Autodesk Inventor part; units mm, degrees
ref_plane "YZ Plane" through (0, 0, 0) normal (1, 0, 0) x (0, 1, 0)
ref_plane "XZ Plane" through (0, 0, 0) normal (0, 1, 0) x (-1, 0, 0)
ref_plane "XY Plane" through (0, 0, 0) normal (0, 0, 1) x (1, 0, 0)
sketch "Sketch1" plane through (0, 0, 0) normal (0, 1, 0) x (-1, 0, 0)
  line L0 (12.5, -50) -> (-12.5, -50)
  line L1 (-12.5, -50) -> (-12.5, 10)
  line L2 (-12.5, 10) -> (12.5, 10)
  line L3 (12.5, 10) -> (12.5, -50)
  line L4 (12.5, 0) -> (-12.5, 0) construction
  line L5 (0, -50) -> (0, 10) construction
  circle A0 centre (7.5, 0) radius 1.6
  line L6 (12.5, 10) -> (146.5, 10)
  line L7 (146.5, 10) -> (146.5, -10)
  line L8 (146.5, -10) -> (12.5, -10)
  line L9 (12.5, -10) -> (12.5, 10)
  line L10 (146.5, 0) -> (12.5, 0) construction
  circle A1 centre (132.7538, 0) radius 2.5
  circle A2 centre (-7.5, 0) radius 1.6
  line L11 (12.5, -40) -> (-12.5, -40) construction
  circle A3 centre (7.5, -40) radius 2.5
  circle A4 centre (-7.5, -40) radius 2.5
  point P0 (0, 0)
  point P1 (0, 0)
  point P2 (12.5, -10)
  dimension "d0" = 3.2
  dimension "d1" = 15
  dimension "d3" = 10
  dimension "d4" = 60
  dimension "d5" = 25
  dimension "d6" = 134
  dimension "d7" = 20
  dimension "d8" = 5
  dimension "d9" = 10
  dimension "d10" = 5
  dimension "d11" = 15
extrude "Extrusion1" add sketch "Sketch1" along normal blind 4
sketch "Sketch2" plane through (0, 0, 0) normal (0, -1, 0) x (1, 0, 0)
  line L0 (-146.5, 10) -> (12.5, 10)
  line L1 (-146.5, -10) -> (-146.5, 10)
  line L2 (-12.5, -10) -> (-146.5, -10)
  line L3 (-12.5, -50) -> (-12.5, -10)
  line L4 (12.5, -50) -> (-12.5, -50)
  line L5 (12.5, 10) -> (12.5, -50)
  circle A0 centre (-7.5, 0) radius 1.6
  circle A1 centre (7.5, 0) radius 1.6
  circle A2 centre (-7.5, -40) radius 2.5
  circle A3 centre (7.5, -40) radius 2.5
  circle A4 centre (-132.7538, 0) radius 2.5
extrude "Extrusion2" add sketch "Sketch2" along normal blind 1 contours L0 L5 L4 L3 L2 L1 | A2 | A3 | A4
properties part number "y_axis_extensor"
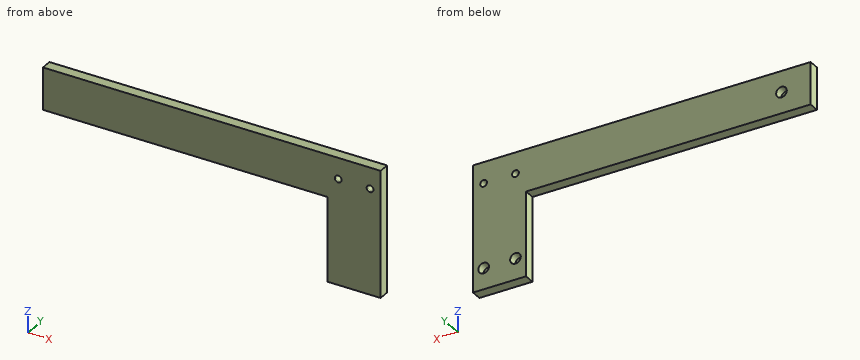
Source: CAD feature listing. Evaluate the final solid. Frame: model axes, mm. Coordinates: 2 decimals unless noted, no trailing zeros. Loops run counter-clockwise (first coordinate to the right, second up) from the corner with the lowest first, then second, coordinate; pieces in that order, holes last. Notation, with made-up numbers: M 30.25,62.25 L 35.25,62.25 A21 ccw 35.25,90.25 Z; hole C -19.75,-35 d5. An arc over 180 degrees is marked long. Answer in a Markdown table with one row per item.
Q1. Section A-A on y = 1.2. Return the cut outline in (x, z).
Answers below:
| item | result |
|---|---|
| outline | M -146.5,-10 L -12.5,-10 L -12.5,-50 L 12.5,-50 L 12.5,10 L -146.5,10 Z; hole C -132.75,0 d5; hole C -7.5,-40 d5; hole C -7.5,0 d3.2; hole C 7.5,-40 d5; hole C 7.5,0 d3.2 |
Q2. Ray query, probe 1 along Z at (x, y) = (-7.5, 1.6); probe 2 along X at (y, z) = (-0.5, 0); probe 3 along X at (y, z) = (2.6, -39). Return the intervals inside material, ascending. Write a range as from..to.
Answers below:
| item | result |
|---|---|
| probe 1 | z = -50..-42.5, -37.5..-1.6, 1.6..10 |
| probe 2 | x = -146.5..-9.1, -5.9..5.9, 9.1..12.5 |
| probe 3 | x = -12.5..-9.79, -5.21..5.21, 9.79..12.5 |
Q3. Section D-D on x = -59.5. Return the cut outline in (y, z), plus the area to 3 significant figures.
Answers below:
| item | result |
|---|---|
| outline | M -1,-10 L 4,-10 L 4,10 L -1,10 Z |
| area | 100 mm^2 |
Q4. Section C-C on z = -40. Return the cut outline in (x, y).
Answers below:
| item | result |
|---|---|
| outline | M -12.5,-1 L 12.5,-1 L 12.5,4 L 10,4 L 10,0 L 5,0 L 5,4 L -5,4 L -5,0 L -10,0 L -10,4 L -12.5,4 Z |
Q5. Section B-B on x = -7.5. Return the cut outline in (y, z), plus the area to 3 significant figures.
Answers below:
| item | result |
|---|---|
| outline | M -1,-50 L 4,-50 L 4,-42.5 L 0,-42.5 L 0,-37.5 L 4,-37.5 L 4,-1.6 L -1,-1.6 Z; M -1,1.6 L 4,1.6 L 4,10 L -1,10 Z |
| area | 264 mm^2 |
Q6. First-contact query: pin 1 (4.5 mm diameter, centred on x = -132.75, z = 0, fed in from +Y); pin 2 (5.5 mm diameter, centred on x = 7, z = -39.5, fed in from +Y); pin 3 (1 mm diameter, centred on x = -19, y = 3, fed in from -Z). Flat tips, straight axial feed; report the tip coordinate or a pass-through.
Answers below:
| item | result |
|---|---|
| pin 1 | stops at y = 0 |
| pin 2 | stops at y = 4 |
| pin 3 | stops at z = -10 |
